Here's the drawing with two shaded views (mm, measured from the low corner). I have some questions. Give positions to 0.01 mm unless a question says otherwise; leave off trailing zeros. Write each loop counter-clockwise with the first axis right and the second up, starting at its lowest first coordinate (ties: lowest second). Pieces come first, ordered by that corner, then holes. Notation, with made-up numbers: (71.25, 79.25) - (110.25, 79.25) arc R16 ccw to (110.25, 107.25) - close; hole circle Ø4 at (-15, 1). An arc over 180 degrees is marked (long way). Answer as CSV lines item,"result". Start each with the question number.
Q1. If I drill on line 1 along X through (y, z) = (56.59, 1.1); line 2 along X through (y, z) = (39, 1.2); line 3 along X through (y, z) = (23, 1.9), over which ranges is the centre line in solid material (lowest first)?
Q2. Imagine slicing it at B-B on y = 44.09. List the corners of the cut face in (x, z) for me, and give its area (3 significant figures).
Q3. Imagine slicing it at D-D on y = 12. List the corners of the cut face in (x, z) for me (1 decimal), and give its area (3 significant figures).
Q4. Imagine slicing it at A-A on y = 56.59. List the corners of the cut face in (x, z) for me.
Q5. Imagine slicing it at C-C on z = 1.4. List the corners of the cut face in (x, y) for me, and give its area (3 significant figures).
Q6. Will these pins go through, and if not, where does the flat tip stop? pin 1 Ø8 at (x, y) = (21, 51) entering from -Z; pin 2 Ø3 at (x, y) = (39.5, 24.09) entering from -Z; pin 3 Ø1.2 at (y, z) = (47.5, 1.5) entering from -X; pin 4 Ø0.8 at (x, z) = (77.5, 1) entering from -Y.
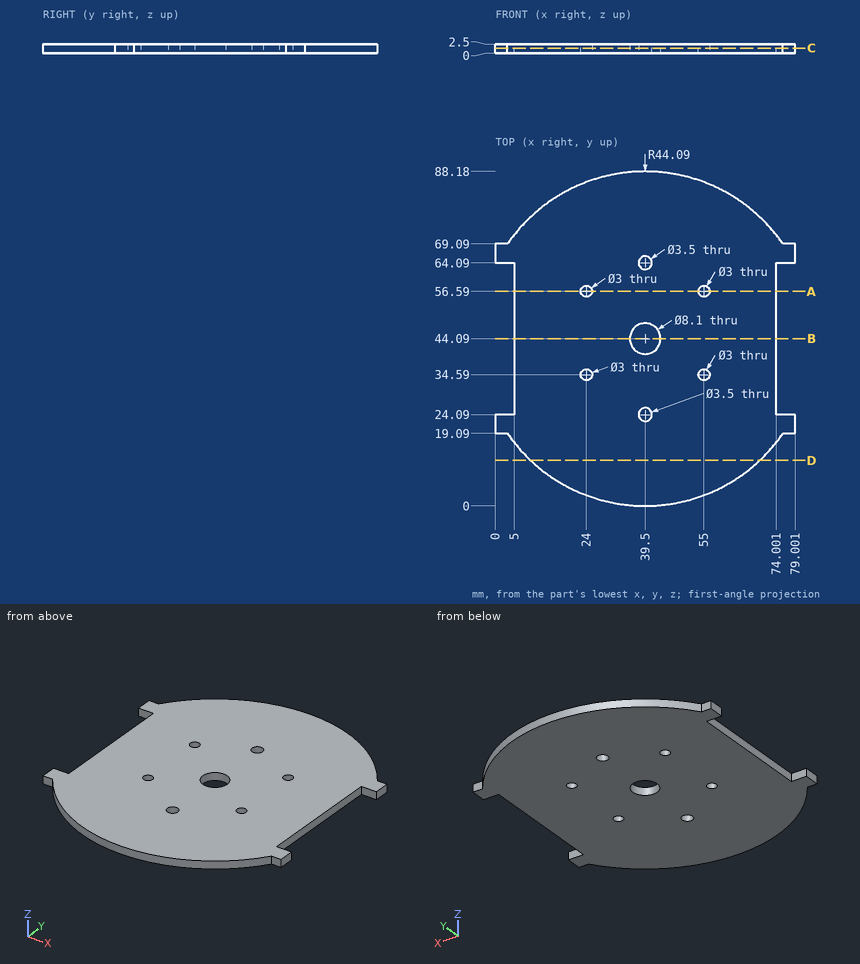
Conclusion:
1,line 1,"5 to 22.5, 25.5 to 53.5, 56.5 to 74"
1,line 2,"5 to 74"
1,line 3,"0 to 38.13, 40.87 to 79"
2,outline,"(5, 0) - (35.45, 0) - (35.45, 2.5) - (5, 2.5) - close; (43.55, 0) - (74, 0) - (74, 2.5) - (43.55, 2.5) - close"
2,area,"152 mm^2"
3,outline,"(9.3, 0) - (69.7, 0) - (69.7, 2.5) - (9.3, 2.5) - close"
3,area,"151 mm^2"
4,outline,"(5, 0) - (22.5, 0) - (22.5, 2.5) - (5, 2.5) - close; (25.5, 0) - (53.5, 0) - (53.5, 2.5) - (25.5, 2.5) - close; (56.5, 0) - (74, 0) - (74, 2.5) - (56.5, 2.5) - close"
5,outline,"(0, 19.09) - (3.18, 19.09) arc R44.09 ccw to (75.82, 19.09) - (79, 19.09) - (79, 24.09) - (74, 24.09) - (74, 64.09) - (79, 64.09) - (79, 69.09) - (75.82, 69.09) arc R44.09 ccw to (3.18, 69.09) - (0, 69.09) - (0, 64.09) - (5, 64.09) - (5, 24.09) - (0, 24.09) - close; hole circle Ø3 at (24, 34.59); hole circle Ø3 at (24, 56.59); hole circle Ø8.1 at (39.5, 44.09); hole circle Ø3.5 at (39.5, 24.09); hole circle Ø3.5 at (39.5, 64.09); hole circle Ø3 at (55, 34.59); hole circle Ø3 at (55, 56.59)"
5,area,"5,400 mm^2"
6,pin 1,"z = 0"
6,pin 2,"through"
6,pin 3,"x = 5"
6,pin 4,"y = 19.09"
